from build123d import *

# Parameters (mm, degrees)
SKETCH2_W           = 10
SKETCH2_H           = 14.768412439
BOSS_EXTRUDE1_DEPTH = 5
BOSS_EXTRUDE4_DEPTH = 10
SKETCH9_W           = 10
SKETCH9_H           = 3.18
SKETCH9_H_2         = 3.888412439
CUT_EXTRUDE3_DEPTH  = 5
BOSS_EXTRUDE5_DEPTH = 7.7
SKETCH12_R          = 0.75
BOSS_EXTRUDE7_DEPTH = 2.75
FILLET1_R           = 2.5
SKETCH13_W          = 17.887250462
SKETCH13_H          = 46.229219396
CUT_EXTRUDE4_DEPTH  = 20
SKETCH15_W          = 10
SKETCH15_H          = 7.7
BOSS_EXTRUDE9_DEPTH = 100
CUT_EXTRUDE5_DEPTH  = 100


with BuildPart() as part:
    # Sketch2 → Boss-Extrude1 (new body)
    with BuildSketch(Plane.XY):
        with Locations((0, 1.566049366)):
            Rectangle(SKETCH2_W, SKETCH2_H)
    extrude(amount=BOSS_EXTRUDE1_DEPTH)

    # Sketch8 → Boss-Extrude4 (add)
    with BuildSketch(Plane.ZY.offset(5)):
        Polygon((-0.15, 5.770255585), (0, 5.770255585), (0, 4.070255585), (-0.15, 4.070255585), (-2.137867966, 4.070255585), (-3.402081528, 5.334469147), (-2.2, 6.536550675), (-1.43370491, 5.770255585), align=None)
        Polygon((-0.15, -1.929744415), (0, -1.929744415), (0, -0.229744415), (-0.15, -0.229744415), (-1.43370491, -0.229744415), (-2.2, 0.536550675), (-3.402081528, -0.665530853), (-2.137867966, -1.929744415), align=None)
    extrude(amount=-BOSS_EXTRUDE4_DEPTH)

    # Sketch9 → Cut-Extrude3 (cut)
    with BuildSketch(Plane(origin=(0, 0, 0), x_dir=(-1, 0, 0), z_dir=(0, 0, -1))):
        with Locations((0, 7.360255585)):
            Rectangle(SKETCH9_W, SKETCH9_H)
        with Locations((0, -3.873950635)):
            Rectangle(SKETCH9_W, SKETCH9_H_2)
    extrude(amount=-CUT_EXTRUDE3_DEPTH, mode=Mode.SUBTRACT)

    # Sketch10 → Boss-Extrude5 (add)
    with BuildSketch(Plane(origin=(0, 5.770255585, 0), x_dir=(1, 0, 0), z_dir=(0, 1, 0))):
        with BuildLine():
            Line((-5, -5), (-5, -10.5))
            Line((-5, -10.5), (1.352445729, -55.7))
            Line((1.352445729, -55.7), (6.352445729, -55.7))
            Line((6.352445729, -55.7), (6.352445729, -49.2))
            ThreePointArc((6.352445729, -49.2), (1.383429579, -31.764936646), (5, -14))
            Line((5, -14), (5, -5))
            Line((5, -5), (-5, -5))
        make_face()
    extrude(amount=-BOSS_EXTRUDE5_DEPTH)

    # Sketch12 → Boss-Extrude7 (add)
    with BuildSketch(Plane.XY):
        with BuildLine():
            Line((5, 5.770255585), (8.5, 5.770255585))
            ThreePointArc((8.5, 5.770255585), (12.35, 1.920255585), (8.5, -1.929744415))
            Line((8.5, -1.929744415), (5, -1.929744415))
            Line((5, -1.929744415), (5, 5.770255585))
        make_face()
        with Locations((8.5, 1.920255585)):
            Circle(SKETCH12_R, mode=Mode.SUBTRACT)
    extrude(amount=BOSS_EXTRUDE7_DEPTH)

    # Fillet1
    fillet1_edges = [part.edges().sort_by_distance(p)[0] for p in [
        (6.352445729, 1.920255585, 49.2),
        (5, 1.920255585, 14),
        (1.352445729, 1.920255585, 55.7),
        (6.352445729, 1.920255585, 55.7),
    ]]
    fillet(fillet1_edges, radius=FILLET1_R)

    # Sketch13 → Cut-Extrude4 (cut)
    with BuildSketch(Plane(origin=(0, 5.770255585, 0), x_dir=(1, 0, 0), z_dir=(0, 1, 0))):
        with Locations((3.943625231, -33.614609698)):
            Rectangle(SKETCH13_W, SKETCH13_H)
    extrude(amount=-CUT_EXTRUDE4_DEPTH, mode=Mode.SUBTRACT)

    # Sketch15 → Boss-Extrude9 (add)
    with BuildSketch(Plane.XY.offset(10.5)):
        with Locations((0, 1.920255585)):
            Rectangle(SKETCH15_W, SKETCH15_H)
    extrude(amount=BOSS_EXTRUDE9_DEPTH)

    # Sketch16 → Cut-Extrude5 (cut)
    with BuildSketch(Plane(origin=(0, 5.770255585, 0), x_dir=(1, 0, 0), z_dir=(0, 1, 0))):
        Polygon((-5, -7.952810564), (2.461220142, -110.5), (-5, -110.5), align=None)
    extrude(amount=-CUT_EXTRUDE5_DEPTH, mode=Mode.SUBTRACT)


solid = part.part
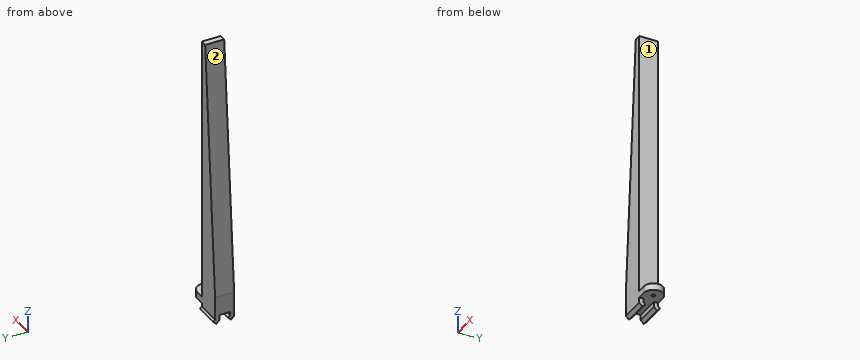
Here's how the part is built. I have some questions about the finished solid (model axes, mm). Face numbers are marked on the shaded views. A direction names the side the tool comes from. Coordinates: 2 decimals unless noted, no trailing zeros. Write each loop counter-clockwise with the first axis right and the second up, starting at its lowest first coordinate (ties: lowest second). Pieces come first, ordered by that corner, then holes.
Item 1: Will these pins go through, and if not, where does the flat tip stop? pin 1 (7 mm diameter, centred on x = 2.5, z = 71, fed in from +Y); pin 2 (1.2 mm diameter, centred on y = -1.5, z = -2, fed in from +X); pin 3 (1.2 mm diameter, centred on x = 8.5, y = 1.92, fed in from +Z); pin 4 (4 mm diameter, centred on x = 8, y = 2, fed in from -Z).
Item 2: If I drill on line 1 (Y direction, x = 8.5, z = 0.85); line 2 (X direction, y = 2, z = 2); line 3 (Z direction, x = 9.25, y = -1.25), over which ranges is the centre line in solid material (lowest first)?
Item 3: I want a section at B-B on z = 70.5. Write out the boundary of the cut face in (x, y).
Item 4: I want a section at C-C on z = 88. Write out the boundary of the cut face in (x, y).
Item 5: On a 3-axis mill with a long thin cutter (end or side, diameter ignored), from which of +Z, -Z, +X, -X, +Y, -Y can I reach the whole of each face in a straight line? I mean the marked faces 1 and 2. Say none if no direction works.
Item 6: I want a section at A-A on x = -1.25. Write out the boundary of the cut face in (y, z).
Findings below:
1. pin 1: stops at y = 5.77
1. pin 2: stops at x = 5
1. pin 3: passes through
1. pin 4: stops at z = 0
2. line 1: y = -1.93 to 1.17, 2.67 to 5.77
2. line 2: x = -5 to 7.75, 9.25 to 12.35
2. line 3: z = 0 to 2.75
3. outline: (-0.45, -1.93) - (5, -1.93) - (5, 5.77) - (-0.45, 5.77) - close
4. outline: (0.82, -1.93) - (5, -1.93) - (5, 5.77) - (0.82, 5.77) - close
5. face 1: +Z, +X, +Y, -Y
5. face 2: +Z, -X, +Y, -Y
6. outline: (-1.93, -2.14) - (-0.67, -3.4) - (0.54, -2.2) - (-0.23, -1.43) - (-0.23, 0) - (4.07, 0) - (4.07, -2.14) - (5.33, -3.4) - (6.54, -2.2) - (5.77, -1.43) - (5.77, 59.49) - (-1.93, 59.49) - close
